from build123d import *

# Parameters (mm, degrees)
SKETCH1_W               = 11.811
SKETCH1_H               = 45.98924
BOSS_EXTRUDE1_DEPTH     = 9.652
FILLET5_R               = 4.826
SKETCH2_W               = 7.62
SKETCH2_H               = 22.352
CUT_EXTRUDE1_DEPTH      = 7.62
CUT_EXTRUDE2_DEPTH      = 49.452771033
CUT_EXTRUDE2_DEPTH_BACK = 49.452771033
SKETCH3_R               = 2.20345
FILLET4_R               = 4.826
FILLET6_R               = 10.16
CUT_EXTRUDE3_DEPTH      = 49.452771033
CUT_EXTRUDE4_DEPTH      = 7.62
BOSS_EXTRUDE2_DEPTH     = 7.62


with BuildPart() as part:
    # Sketch1 → Boss-Extrude1 (new body)
    with BuildSketch(Plane.XY):
        with Locations((5.9055, 22.99462)):
            Rectangle(SKETCH1_W, SKETCH1_H)
    extrude(amount=BOSS_EXTRUDE1_DEPTH)

    # Fillet5
    fillet5_edges = [part.edges().sort_by_distance(p)[0] for p in [
        (5.9055, 45.98924, 0),
    ]]
    fillet(fillet5_edges, radius=FILLET5_R)

    # Sketch2 → Cut-Extrude1 (cut)
    with BuildSketch(Plane(origin=(0, 0, 0), x_dir=(-1, 0, 0), z_dir=(0, 0, -1))):
        with Locations((-5.9055, 34.81324)):
            Rectangle(SKETCH2_W, SKETCH2_H)
    extrude(amount=-CUT_EXTRUDE1_DEPTH, mode=Mode.SUBTRACT)

    # Sketch3 → Cut-Extrude2 (cut, two sides: drawn at the far end of the back side and taken through both)
    with BuildSketch(Plane.ZY.offset(-CUT_EXTRUDE2_DEPTH_BACK)):
        with Locations((4.4323, 26.82494)):
            Circle(SKETCH3_R)
    extrude(amount=CUT_EXTRUDE2_DEPTH + CUT_EXTRUDE2_DEPTH_BACK, mode=Mode.SUBTRACT)

    # Fillet4
    # the kernel refuses this fillet: 4.826 mm, written as the material it takes off along each edge
    with BuildSketch(Plane(origin=(23.876, 45.98924, 9.652), x_dir=(0, 0, -1), z_dir=(-1, 0, 0))) as fillet4_piece_1:
        with BuildLine():
            CenterArc((FILLET4_R, FILLET4_R), FILLET4_R, 180, 90)
            Line((0, FILLET4_R), (0, 0))
            Line((0, 0), (FILLET4_R, 0))
        make_face()
    extrude(amount=35.941, mode=Mode.SUBTRACT)

    # Fillet6
    # the kernel refuses this fillet: 10.16 mm, written as the material it takes off along each edge
    with BuildSketch(Plane(origin=(-25.368230131, 0, 9.652), x_dir=(0, 1, 0), z_dir=(1, 0, 0))) as fillet6_piece_1:
        with BuildLine():
            CenterArc((10.147292053, -10.16), FILLET6_R, 90, 87.134016017)
            Line((0, -9.652), (-0.202945841, -9.64184))
            ThreePointArc((-0.202945841, -9.64184), (-0.2032, -4.826), (-0.2032, 0))
            Line((-0.2032, 0), (0, 0.2032))
            Line((0, 0.2032), (10.147292053, 0.2032))
            Line((10.147292053, 0.2032), (10.147292053, 0))
        make_face()
    extrude(amount=62.547460263, mode=Mode.SUBTRACT)

    # Sketch4 → Cut-Extrude3 (cut, through all)
    with BuildSketch(Plane(origin=(11.811, 0, 0), x_dir=(0, 0, -1), z_dir=(1, 0, 0))):
        Polygon((-9.652, 26.403813088), (-7.62, 30.63494), (0, 30.63494), (0, 45.98924), (-9.652, 45.98924), align=None)
    extrude(amount=-CUT_EXTRUDE3_DEPTH, mode=Mode.SUBTRACT)

    # Sketch5 → Cut-Extrude4 (cut)
    with BuildSketch(Plane.ZY.offset(-9.7155)):
        Polygon((0, 21.160076085), (5.158068358, 23.63724), (0, 23.63724), align=None)
    extrude(amount=CUT_EXTRUDE4_DEPTH, mode=Mode.SUBTRACT)

    # Sketch5<3> → Boss-Extrude2 (add)
    with BuildSketch(Plane.ZY.offset(-9.7155)):
        with BuildLine():
            Line((5.812301369, 23.951435604), (5.158068358, 23.63724))
            Line((5.158068358, 23.63724), (7.62, 23.63724))
            Line((7.62, 23.63724), (7.62, 26.82494))
            ThreePointArc((7.62, 26.82494), (7.130490287, 25.127530072), (5.812301369, 23.951435604))
        make_face()
    extrude(amount=BOSS_EXTRUDE2_DEPTH)


solid = part.part
Work out the finished part from the listing and answer in its coordinate system (mm). A direction names the side the tool comes from. Give positions to 0.01 mm unless a question says otherwise; leave off trailing zeros. Write each loop counter-clockwise with the first axis right and the second up, starting at its lowest first coordinate (ties: lowest second). Pieces come first, ordered by that corner, then holes.
Q1. The part is cut by section D-D on z = 7.25. Give the vertices of the cut face in (x, y).
Answer:
outline: (0, 3.59) - (11.81, 3.59) - (11.81, 30.63) - (9.72, 30.63) - (9.72, 25.33) - (2.1, 25.33) - (2.1, 30.63) - (0, 30.63) - close
Q2. For a pull along X with two mould halves and no side action, classify faces 1 (the face through (11.811, 15, 5)), 2 (the face through (5.959, 25.149, 7.144)), 3 (the face through (0, 15, 5)), 4 (the face through (11, 30.635, 4)) as released by +X, released by -X, zero draft, split by the parting line, or undercut.
Answer:
face 1: released by +X
face 2: undercut
face 3: released by -X
face 4: zero draft
Q3. Given pin 1 (2 mm diameter, centred on x = 9.5, z = 5.5, fed in from -Y); pin 2 (3 mm diameter, centred on x = 5, y = 29.5, fed in from -Z); pin 3 (1.5 mm diameter, centred on x = 5.5, z = 3.5, fed in from -Y), each flat-ended and moving along its own axis, determine where each tip first touches the part or whether it passes through.
Answer:
pin 1: stops at y = 1.31
pin 2: stops at z = 7.62
pin 3: stops at y = 0.52
Q4. The part is cut by section B-B on x = 6.75. Give the vertices of the cut face in (y, z).
Answer:
outline: (0, 0) - (21.16, 0) - (23.95, 5.81) arc R3.19 cw to (26.82, 7.62) - (30.63, 7.62) - (26.4, 9.65) - (10.15, 9.65) arc R10.16 ccw to start
Q5. A tool of negligible diameter and unlimited length cuts with its end or side. For faces 5 (the face through (2.096, 27, 2)), 6 (the face through (5.99, 28.49, 8.65)), from which of +Z, -Z, +X, -X, +Y, -Y can it reach the whole face along a straight path? Write none if from no direction.
Answer:
face 5: -Z, +Y
face 6: +Z, +X, -X, +Y
Q6. Straight lines are drawn through the part: L1, parallel to X at y = 29.5, z = 4.5; L2, parallel to Y at x = 7, z = 2.25; L3, parallel to Z at x = 1.5, y = 27.5. For each, find the intervals that lie inside material, in ascending order.
Answer:
L1: x = 0 to 2.1, 9.72 to 11.81
L2: y = 0.37 to 22.24
L3: z = 0 to 2.33, 6.53 to 9.13
Q7. The part is cut by section A-A on z = 4.25. Give the vertices of the cut face in (x, y), and give its area (3 significant figures).
Answer:
outline: (0, 1.17) - (11.81, 1.17) - (11.81, 24.63) - (9.72, 24.63) - (9.72, 23.2) - (2.1, 23.2) - (2.1, 24.63) - (0, 24.63) - close; (0, 29.02) - (2.1, 29.02) - (2.1, 30.63) - (0, 30.63) - close; (9.72, 29.02) - (11.81, 29.02) - (11.81, 30.63) - (9.72, 30.63) - close
area: 273 mm2
Q8. The part is cut by section C-C on x = 10.25. Give the vertices of the cut face in (y, z), and give its area (3 significant figures).
Answer:
outline: (0, 0) - (30.63, 0) - (30.63, 7.62) - (26.4, 9.65) - (10.15, 9.65) arc R10.16 ccw to start; hole circle Ø4.41 at (26.82, 4.43)
area: 254 mm2
